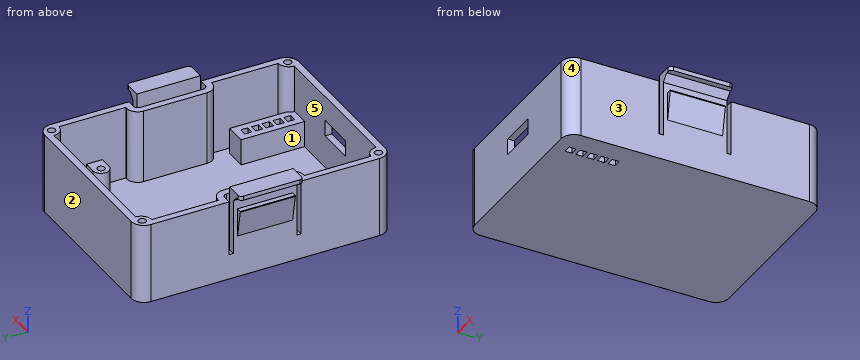
from build123d import *

# Parameters (mm, degrees)
SKETCH_1_W               = 44
SKETCH_1_H               = 60
EXTRUDE_1_DEPTH          = 19
SKETCH_2_W               = 3
SKETCH_2_H               = 17
CUT_EXTRUDE_1_DEPTH      = 42.773197148
FILLET_1_R               = 3
FILLET_2_R               = 1
SHELL_1_T                = -1.6
EXTRUDE_2_DEPTH          = 17.4
SKETCH_3_3_R             = 0.9
CUT_EXTRUDE_2_DEPTH      = 17.4
MIRROR_2_COPY_1_DEPTH    = 17.4
MIRROR_2_COPY_2_SKETCH_R = 0.9
MIRROR_2_COPY_2_DEPTH    = 17.4
SKETCH_4_W               = 5
SKETCH_4_H               = 15
EXTRUDE_3_DEPTH          = 6.2
CUT_EXTRUDE_3_DEPTH      = 42.070183832
CUT_EXTRUDE_3_DEPTH_BACK = 42.070183832
SKETCH_4_4_W             = 1.8
SKETCH_4_4_H             = 1.7
SKETCH_5_R               = 0.9
EXTRUDE_4_DEPTH          = 6.2
SKETCH_6_W               = 9
SKETCH_6_H               = 3.8
CUT_EXTRUDE_4_DEPTH      = 66.234653368
SKETCH_8_W               = 3
SKETCH_8_H               = 17
EXTRUDE_5_DEPTH          = 6
SKETCH_9_W               = 1.6
SKETCH_9_H               = 15
EXTRUDE_6_DEPTH          = 15.5
EXTRUDE_7_DEPTH          = 15
EXTRUDE_8_DEPTH          = 6.5
FILLET_3_R               = 0.8
FILLET_3_OF_MIRROR_3_R   = 0.8


with BuildPart() as part:
    # 草图1 → 凸台-拉伸1 (new body)
    with BuildSketch(Plane.XY):
        Rectangle(SKETCH_1_W, SKETCH_1_H)
    extrude(amount=EXTRUDE_1_DEPTH)

    # 草图2 → 切除-拉伸1 (cut, through all)
    with BuildSketch(Plane.XY.offset(19)):
        with Locations((-20.5, 0)):
            Rectangle(SKETCH_2_W, SKETCH_2_H)
        with Locations((20.5, 0)):
            Rectangle(SKETCH_2_W, SKETCH_2_H)
    extrude(amount=-CUT_EXTRUDE_1_DEPTH, mode=Mode.SUBTRACT)

    # 圆角1
    fillet_1_edges = [part.edges().sort_by_distance(p)[0] for p in [
        (22, -30, 9.5),
        (-22, -30, 9.5),
        (-22, 30, 9.5),
        (22, 30, 9.5),
    ]]
    fillet(fillet_1_edges, radius=FILLET_1_R)

    # 圆角2
    fillet_2_edges = [part.edges().sort_by_distance(p)[0] for p in [
        (-19, 8.5, 9.5),
        (-19, -8.5, 9.5),
        (19, -8.5, 9.5),
        (19, 8.5, 9.5),
    ]]
    fillet(fillet_2_edges, radius=FILLET_2_R)

    # 抽壳1
    shell_1_openings = [part.faces().sort_by_distance(p)[0] for p in [
        (0, 0, 19),
    ]]
    offset(amount=SHELL_1_T, openings=shell_1_openings, kind=Kind.INTERSECTION)

    # 草图3 → 凸台-拉伸2 (add)
    with BuildSketch(Plane.XY.offset(1.6)):
        with BuildLine():
            Line((-20.4, 28.4), (-17.9, 28.4))
            ThreePointArc((-17.9, 28.4), (-18.632233047, 26.632233047), (-20.4, 25.9))
            Line((-20.4, 25.9), (-20.4, 28.4))
        make_face()
    extrude_2 = extrude(amount=EXTRUDE_2_DEPTH)

    # 草图3<3> → 切除-拉伸2 (cut)
    with BuildSketch(Plane.XY.offset(1.6)):
        with Locations(Location((-19.9, 27.9, 0), (0, 0, 180))):
            Circle(SKETCH_3_3_R)
    cut_extrude_2 = extrude(amount=CUT_EXTRUDE_2_DEPTH, mode=Mode.SUBTRACT)

    # 镜向1: 凸台-拉伸2, 切除-拉伸2 across plane
    add(extrude_2.mirror(Plane(origin=(0, 0, 0), x_dir=(0, 0, 1), z_dir=(1, 0, 0))))
    add(cut_extrude_2.mirror(Plane(origin=(0, 0, 0), x_dir=(0, 0, 1), z_dir=(1, 0, 0))), mode=Mode.SUBTRACT)

    # 镜向2: 凸台-拉伸2, 切除-拉伸2 across plane
    add(extrude_2.mirror(Plane.ZX))
    add(cut_extrude_2.mirror(Plane.ZX), mode=Mode.SUBTRACT)

    # 镜向2 copy 1 sketch → 镜向2 copy 1 (add)
    with BuildSketch(Plane(origin=(0, 0, 1.6), x_dir=(-1, 0, 0), z_dir=(0, 0, 1))):
        with BuildLine():
            Line((-20.4, 28.4), (-17.9, 28.4))
            ThreePointArc((-17.9, 28.4), (-18.632233047, 26.632233047), (-20.4, 25.9))
            Line((-20.4, 25.9), (-20.4, 28.4))
        make_face()
    extrude(amount=MIRROR_2_COPY_1_DEPTH)

    # 镜向2 copy 2 sketch → 镜向2 copy 2 (cut)
    with BuildSketch(Plane(origin=(0, 0, 1.6), x_dir=(-1, 0, 0), z_dir=(0, 0, 1))):
        with Locations(Location((-19.9, 27.9, 0), (0, 0, 180))):
            Circle(MIRROR_2_COPY_2_SKETCH_R)
    extrude(amount=MIRROR_2_COPY_2_DEPTH, mode=Mode.SUBTRACT)

    # 草图4 → 凸台-拉伸3 (add)
    with BuildSketch(Plane.XY.offset(1.6)):
        with Locations((16, -20.9)):
            Rectangle(SKETCH_4_W, SKETCH_4_H)
    extrude(amount=EXTRUDE_3_DEPTH)

    # 草图4<4> → 切除-拉伸3 (cut, two sides: drawn at the far end of the back side and taken through both)
    with BuildSketch(Plane.XY.offset(1.6).offset(-CUT_EXTRUDE_3_DEPTH_BACK)):
        with Locations((16, -26.15)):
            Rectangle(SKETCH_4_4_W, SKETCH_4_4_H)
        with Locations((16, -23.61)):
            Rectangle(SKETCH_4_4_W, SKETCH_4_4_H)
        with Locations((16, -21.07)):
            Rectangle(SKETCH_4_4_W, SKETCH_4_4_H)
        with Locations((16, -18.53)):
            Rectangle(SKETCH_4_4_W, SKETCH_4_4_H)
        with Locations((16, -15.99)):
            Rectangle(SKETCH_4_4_W, SKETCH_4_4_H)
    extrude(amount=CUT_EXTRUDE_3_DEPTH + CUT_EXTRUDE_3_DEPTH_BACK, mode=Mode.SUBTRACT)

    # 草图5 → 凸台-拉伸4 (add)
    # profile 1 of 3: a face of its own
    with BuildSketch(Plane.XY.offset(1.6)):
        with BuildLine():
            Line((-17.5, 19.4), (-20.4, 19.4))
            Line((-20.4, 19.4), (-20.4, 15.6))
            Line((-20.4, 15.6), (-17.5, 15.6))
            ThreePointArc((-17.5, 15.6), (-15.6, 17.5), (-17.5, 19.4))
        make_face()
        with Locations(Location((-17.5, 17.5, 0), (0, 0, 180))):
            Circle(SKETCH_5_R, mode=Mode.SUBTRACT)
    # profile 2 of 3: a face of its own
    with BuildSketch(Plane.XY.offset(1.6)):
        with BuildLine():
            Line((20.4, 15.6), (17.5, 15.6))
            ThreePointArc((17.5, 15.6), (15.6, 17.5), (17.5, 19.4))
            Line((17.5, 19.4), (20.4, 19.4))
            Line((20.4, 19.4), (20.4, 15.6))
        make_face()
        with Locations(Location((17.5, 17.5, 0), (0, 0, 180))):
            Circle(SKETCH_5_R, mode=Mode.SUBTRACT)
    # profile 3 of 3: a face of its own
    with BuildSketch(Plane.XY.offset(1.6)):
        with BuildLine():
            Line((-20.4, -15.6), (-17.5, -15.6))
            ThreePointArc((-17.5, -15.6), (-15.6, -17.5), (-17.5, -19.4))
            Line((-17.5, -19.4), (-20.4, -19.4))
            Line((-20.4, -19.4), (-20.4, -15.6))
        make_face()
        with Locations(Location((-17.5, -17.5, 0), (0, 0, 180))):
            Circle(SKETCH_5_R, mode=Mode.SUBTRACT)
    extrude(amount=EXTRUDE_4_DEPTH)

    # 草图6 → 切除-拉伸4 (cut, through all)
    with BuildSketch(Plane(origin=(0, -28.4, 0), x_dir=(1, 0, 0), z_dir=(0, 1, 0))):
        with Locations((0, -11.2)):
            Rectangle(SKETCH_6_W, SKETCH_6_H)
    extrude(amount=-CUT_EXTRUDE_4_DEPTH, mode=Mode.SUBTRACT)

    # 草图8 → 凸台-拉伸5 (add)
    with BuildSketch(Plane(origin=(0, 0, 0), x_dir=(-1, 0, 0), z_dir=(0, 0, -1))):
        with Locations((-20.5, 0)):
            Rectangle(SKETCH_8_W, SKETCH_8_H)
    extrude_5 = extrude(amount=-EXTRUDE_5_DEPTH)

    # 草图9 → 凸台-拉伸6 (add)
    with BuildSketch(Plane.XY.offset(6)):
        with Locations((21.2, 0)):
            Rectangle(SKETCH_9_W, SKETCH_9_H)
    extrude_6 = extrude(amount=EXTRUDE_6_DEPTH)

    # 草图10 → 凸台-拉伸7 (add)
    with BuildSketch(Plane.XZ.offset(7.5)):
        Polygon((22, 21.5), (24.9, 21.5), (24.9, 20.5), (23.5, 20.5), (22, 19), align=None)
    extrude_7 = extrude(amount=-EXTRUDE_7_DEPTH)

    # 草图11 → 凸台-拉伸8 (add, symmetric)
    with BuildSketch(Plane(origin=(0, 0, 0), x_dir=(1, 0, 0), z_dir=(0, 1, 0))):
        Polygon((23.2, -16.5), (22, -10), (22, -16.7), (23.2, -16.7), align=None)
    extrude_8 = extrude(amount=EXTRUDE_8_DEPTH, both=True)

    # 圆角3
    fillet_3_edges = [part.edges().sort_by_distance(p)[0] for p in [
        (24.9, -7.5, 21),
        (24.9, 7.5, 21),
    ]]
    fillet(fillet_3_edges, radius=FILLET_3_R)

    # 镜向3: 凸台-拉伸5, 凸台-拉伸6, 凸台-拉伸7, 凸台-拉伸8 across plane
    add(extrude_5.mirror(Plane(origin=(0, 0, 0), x_dir=(0, 0, 1), z_dir=(1, 0, 0))))
    add(extrude_6.mirror(Plane(origin=(0, 0, 0), x_dir=(0, 0, 1), z_dir=(1, 0, 0))))
    add(extrude_7.mirror(Plane(origin=(0, 0, 0), x_dir=(0, 0, 1), z_dir=(1, 0, 0))))
    add(extrude_8.mirror(Plane(origin=(0, 0, 0), x_dir=(0, 0, 1), z_dir=(1, 0, 0))))

    # 圆角3 of 镜向3
    fillet_3_of_mirror_3_edges = [part.edges().sort_by_distance(p)[0] for p in [
        (-24.9, -7.5, 21),
        (-24.9, 7.5, 21),
    ]]
    fillet(fillet_3_of_mirror_3_edges, radius=FILLET_3_OF_MIRROR_3_R)


solid = part.part
Work out the finished part from the listing and answer in its coordinate system (mm). Face numbers are marked on the shaded views. A direction names the side the tool comes from. Coordinates: 2 decimals unless noted, no trailing zeros. Write each loop counter-clockwise with the first axis right and the second up, starting at its lowest first coordinate (ties: lowest second). Pieces come first, ordered by that corner, then holes. Notation, with made-up numbers: M -8.5,-40 L -0.5,-40 A27 ccw -0.5,-24 Z; hole C -15,19.5 d7. An arc over 180 degrees is marked long. Answer as CSV lines item,"result". Start each with the question number.
Item 1: Section A-A on z = 19.75 is taken. Write down the section's boundary in (x, y).
Item 2: Section B-B on y = 17.5 is taken. Write down the section's boundary in (x, z).
Item 3: A tool of negligible diameter and unlimited length cuts with its end or side. For the marked faces 1 and 2, from which of +Z, -Z, +X, -X, +Y, -Y can it reach the whole face along a straight path? Write none if from no direction.
Item 4: Determine the mould class of the marked faces 3, 4 and 5 for opening direction Y: released by +Y, released by -Y, zero draft, split by the parting line, or undercut.
Item 5: Consider L1, parallel to X at y = -23, z = 2; L2, parallel to Y at x = 11, z = 5.75; L3, parallel to X at y = 0.5, z = 7.25. Determine where each line is inside the solid, lowest interval first.
Item 6: Section C-C on z = 11.25 is taken. Give the number of separate pieces and of enclosed holes in the cut face, and give its area (3 significant figures).
Item 7: Flat-ended cylindrical pins translate along their axes: P1, Ø1.4, axis at x = 19.5, y = -28.5, coming from the +Z side; P2, Ø0.9, axis at y = -26, z = 5, coming from the +X side; P3, Ø1.4, axis at x = -17, y = 17.5, coming from the +Z side. Find the tip coordinate at first contact, or state that the pin passes through.
Checks:
1,outline,"M -22.75,-7.5 L -20.4,-7.5 L -20.4,7.5 L -22.75,7.5 Z; M 20.4,-7.5 L 22.75,-7.5 L 22.75,7.5 L 20.4,7.5 Z"
2,outline,"M -22,0 L 22,0 L 22,19 L 20.4,19 L 20.4,7.8 L 18.4,7.8 L 18.4,1.6 L 16.6,1.6 L 16.6,7.8 L 15.6,7.8 L 15.6,1.6 L -15.6,1.6 L -15.6,7.8 L -16.6,7.8 L -16.6,1.6 L -18.4,1.6 L -18.4,7.8 L -20.4,7.8 L -20.4,19 L -22,19 Z"
3,face 1,"+Z"
3,face 2,"+Z, -Z, +X, -X, +Y"
4,face 3,"zero draft"
4,face 4,"released by -Y"
4,face 5,"undercut"
5,L1,"x = -22 to -20.4, 13.5 to 15.1, 16.9 to 18.5, 20.4 to 22"
5,L2,"y = -30 to -28.4, 28.4 to 30"
5,L3,"x = -22 to -20.4, -19 to -17.4, 17.4 to 19, 20.4 to 22"
6,separate pieces,"3"
6,enclosed holes,"4"
6,area,"378 mm²"
7,P1,"stops at z = 19"
7,P2,"stops at x = 22"
7,P3,"stops at z = 7.8"
